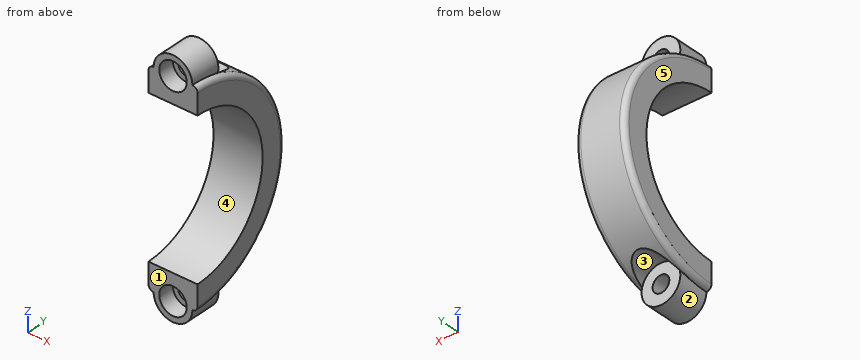
```python
from build123d import *

# Parameters (mm, degrees)
BOSS_EXTRUDE1_DEPTH                               = 12.065
SKETCH2_R                                         = 9.525
BOSS_EXTRUDE2_DEPTH                               = 15.25
CUT_EXTRUDE1_START                                = -15.25
SKETCH2_2_R                                       = 9.525
CUT_EXTRUDE1_DEPTH                                = 15.25
CUT_EXTRUDE1_DRAFT                                = -3
CBORE_FOR_5_16_SOCKET_HEAD_CAP_SCREW1_D           = 8.2042
CBORE_FOR_5_16_SOCKET_HEAD_CAP_SCREW1_CBORE_D     = 13.49502
CBORE_FOR_5_16_SOCKET_HEAD_CAP_SCREW1_CBORE_DEPTH = 7.9375
MIRROR2_START                                     = -15.25
MIRROR2_COPY_1_SKETCH_R                           = 9.525
MIRROR2_COPY_1_DEPTH                              = 15.25
MIRROR2_COPY_1_DRAFT                              = -3
FILLET1_R                                         = 2.54


with BuildPart() as part:
    # Sketch1 → Boss-Extrude1 (new, symmetric)
    with BuildSketch(Plane(origin=(0, 0, 0), x_dir=(0, 0, -1), z_dir=(1, 0, 0))):
        with BuildLine():
            Line((-50.8, 0), (-38.1, 0))
            ThreePointArc((-38.1, 0), (0, 38.1), (38.1, 0))
            Line((38.1, 0), (50.8, 0))
            ThreePointArc((50.8, 0), (0, 50.8), (-50.8, 0))
        make_face()
    extrude(amount=BOSS_EXTRUDE1_DEPTH, both=True)

    # Sketch2 → Boss-Extrude2 (add)
    with BuildSketch(Plane.XZ):
        with Locations((0, -50.8)):
            Circle(SKETCH2_R)
    boss_extrude2 = extrude(amount=-BOSS_EXTRUDE2_DEPTH)


with BuildPart() as cut_extrude1_tool:
    # Sketch2<2> → Cut-Extrude1 (with draft: the straight prism first)
    with BuildSketch(Plane.XZ.offset(CUT_EXTRUDE1_START)):
        with Locations((0, -50.8)):
            Circle(SKETCH2_2_R)
    extrude(amount=-CUT_EXTRUDE1_DEPTH)
    # Cut-Extrude1: the draft: its side faces are tilted about the plane it starts from
    cut_extrude1_sides = [cut_extrude1_tool.faces().sort_by_distance(p)[0] for p in [
        (-9.525, 22.875, -50.8),
    ]]
    draft(cut_extrude1_sides, Plane.XZ.offset(CUT_EXTRUDE1_START), CUT_EXTRUDE1_DRAFT)


with BuildPart() as part_1:
    add(part.part)

    # Cut-Extrude1: cut by cut_extrude1_tool
    add(cut_extrude1_tool.part, mode=Mode.SUBTRACT)

    # CBORE for 5/16 Socket Head Cap Screw1 (through all)
    with Locations(Plane(origin=(0, 0, 0), x_dir=(-1, 0, 0), z_dir=(0, -1, 0))):
        with Locations((0, 50.8)):
            cbore_for_5_16_socket_head_cap_screw1 = CounterBoreHole(CBORE_FOR_5_16_SOCKET_HEAD_CAP_SCREW1_D / 2, CBORE_FOR_5_16_SOCKET_HEAD_CAP_SCREW1_CBORE_D / 2, CBORE_FOR_5_16_SOCKET_HEAD_CAP_SCREW1_CBORE_DEPTH)

    # Mirror1: Boss-Extrude2, CBORE for 5/16 Socket Head Cap Screw1 across plane
    add(boss_extrude2.mirror(Plane.XY))
    add(cbore_for_5_16_socket_head_cap_screw1.mirror(Plane.XY), mode=Mode.SUBTRACT)


with BuildPart() as mirror2_copy_1_tool:
    # Mirror2 copy 1 sketch → Mirror2 copy 1 (with draft: the straight prism first)
    with BuildSketch(Plane.XZ.offset(MIRROR2_START)):
        with Locations((0, 50.8)):
            Circle(MIRROR2_COPY_1_SKETCH_R)
    extrude(amount=-MIRROR2_COPY_1_DEPTH)
    # Mirror2 copy 1: the draft: its side faces are tilted about the plane it starts from
    mirror2_copy_1_sides = [mirror2_copy_1_tool.faces().sort_by_distance(p)[0] for p in [
        (-9.525, 22.875, 50.8),
    ]]
    draft(mirror2_copy_1_sides, Plane.XZ.offset(MIRROR2_START), MIRROR2_COPY_1_DRAFT)


with BuildPart() as part_2:
    add(part_1.part)

    # Mirror2 copy 1: cut by mirror2_copy_1_tool
    add(mirror2_copy_1_tool.part, mode=Mode.SUBTRACT)

    # Fillet1
    fillet1_edges = [part_2.edges().sort_by_distance(p)[0] for p in [
        (12.065, 50.8, 0),
        (-12.065, 50.8, 0),
    ]]
    fillet(fillet1_edges, radius=FILLET1_R - 0.0001)  # a hair under: the kernel refuses the full size


solid = part_2.part
```
Here's how the part is built. I have some questions about the finished solid (model axes, mm). Face numbers are marked on the shaded views. A direction names the side the tool comes from. Coordinates: 2 decimals unless noted, no trailing zeros. Order: outer loops, then holes, each group sorted by start corner. A loop starts at its lowest first (then second) coordinate and runs counter-clockwise, first axis right, second up. Notation, with made-up numbers: (81, 18) - (128, 18) arc R14 ccw to (128, 30) - close; hole circle Ø8 at (-0.75, 68). An arc over 180 degrees is marked (long way). One line per question, with ' | ' between items.
(1) Suppose I cut it at B-B on z = 0. List the corners of the cut face in (x, y) for me (3 decimals), and give its area (3 significant figures).
Report:
outline: (-12.065, 38.1) - (12.065, 38.1) - (12.065, 48.26) arc R2.54 ccw to (9.525, 50.8) - (-9.525, 50.8) arc R2.54 ccw to (-12.065, 48.26) - close | area: 304 mm2
(2) Will these pins go through, and if not, where does the flat tip stop? pin 1 (4 mm diameter, centred on x = 8.5, y = 8.5, fed in from -Z); pin 2 (4 mm diameter, centred on x = -7.5, y = 29, fed in from +Z); pin 3 (12 mm diameter, centred on x = 0, z = -50.8, fed in from +Y); pin 4 (7.5 mm diameter, centred on x = 0, z = 50.8, fed in from -Y).
Report:
pin 1: stops at z = -57.76 | pin 2: stops at z = 43.03 | pin 3: stops at y = 15.25 | pin 4: passes through
(3) For the marked faces 1 and 2, which set-ups out of +Z, -Z, +X, -X, +Y, -Y let a thin tool reach every point of the face, with its end or its side?
Report:
face 1: +Z, -Z, +X, -X, -Y | face 2: +Y
(4) Suppose I cut it at A-A on x = 0. State how many separate pieces and enclosed holes the cut face has, and give its area (3 significant figures).
Report:
separate pieces: 3 | enclosed holes: 0 | area: 1,650 mm2
(5) If I drill on L1, parallel to Z at x = 0.25, y = 10.5; L2, parallel to Z at x = 0, y = 4.75 (1 decimal); L3, parallel to X at y = 6, z = -50.8 (1 decimal), over which ranges is the centre line in solid material (lowest first)?
Report:
L1: z = -60.32 to -54.89, -46.71 to -36.62, 36.62 to 46.71, 54.89 to 60.32 | L2: z = -60.3 to -57.5, -44.1 to -37.8, 37.8 to 44.1, 57.5 to 60.3 | L3: x = -9.5 to -6.7, 6.7 to 9.5
(6) If we mould it in two halves opening along Z, with no side actions, what happens to the marked faces 3, 4 and 5? For each: pulls with the +Z half, pulls with the -Z half, needs draft (parallel to the pull), parting line crosses it, or undercut.
Report:
face 3: pulls with the -Z half | face 4: undercut | face 5: needs draft
